```python
from build123d import *

# Parameters (mm, degrees)
F0_R     = 5
F0_R_2   = 4
F1_DEPTH = 2
F0_R_3   = 2.5
F2_DEPTH = 8.1
F0_R_4   = 1
F3_DEPTH = 12.5
F4_DEPTH = 12.5
F6_D     = 2
F6_DEPTH = 4
F6_TIP   = 0.600860619


with BuildPart() as f1:
    # F0 (on Front) → F1 (new body)
    with BuildSketch(Plane.XZ):
        Circle(F0_R)
        Circle(F0_R_2, mode=Mode.SUBTRACT)
    extrude(amount=F1_DEPTH)

    # F0 (on Front) → F2 (join)
    with BuildSketch(Plane.XZ):
        Circle(F0_R_2)
        Circle(F0_R_3, mode=Mode.SUBTRACT)
    extrude(amount=F2_DEPTH)

    # F0 (on Front) → F3 (join)
    with BuildSketch(Plane.XZ):
        Circle(F0_R_3)
        Circle(F0_R_4, mode=Mode.SUBTRACT)
    extrude(amount=F3_DEPTH)

    # F0 (on Front) → F4 (join)
    with BuildSketch(Plane.XZ):
        Circle(F0_R_4)
    extrude(amount=F4_DEPTH)

    # F6
    with Locations(Plane.XZ.offset(12.5)):
        with Locations((0, 0)):
            Hole(F6_D / 2, depth=F6_DEPTH)
            with Locations((0, 0, -(F6_DEPTH + F6_TIP / 2))):  # 118° drill point
                Cone(0, F6_D / 2, F6_TIP, mode=Mode.SUBTRACT)


solid = f1.part
```
CAD build for the part. Positions are in the model's coordinates, mm. A direction names the side the tool comes from. Round coordinates to 2 decimals unless told otherwise and drop trailing zeros. Order: outer loops, then holes, each group sorted by start corner. A loop starts at its lowest first (then second) coordinate and runs counter-clockwise, first axis right, second up. Notation, with made-up numbers: (73, 9.25) -> (86, 9.25) arc R20 ccw to (86, 27.25) -> close; hole circle Ø4 at (-26, -32). An arc over 180 degrees is marked (long way). One line per question, with ' | ' between items.
Q1. Slice it at A-A (x = 3.75). Write the cut outline in (y, z), then the cut area to 3 significant figures.
Completed:
outline: (-8.1, -1.39) -> (-2, -1.39) -> (-2, -3.31) -> (0, -3.31) -> (0, 3.31) -> (-2, 3.31) -> (-2, 1.39) -> (-8.1, 1.39) -> close | area: 30.2 mm^2
Q2. Slice it at C-C (z = -3.75). Write the cut outline in (x, y).
Completed:
outline: (-3.31, -2) -> (-1.39, -2) -> (-1.39, -8.1) -> (1.39, -8.1) -> (1.39, -2) -> (3.31, -2) -> (3.31, 0) -> (-3.31, 0) -> close
Q3. Which spindle directions (+Z, -Z, +X, -X, +Y, -Y) get a long thin tool onto all of the face, cutting with end or side? Do faces 5 (the cylindrical face through (-0.867, -5.007, -3.905)), 6 (the flat face through (0, 0, 0)). Say none if no direction does.
Completed:
face 5: -Y | face 6: +Z, -Z, +X, -X, +Y
Q4. Probe probe 1 along Z at (x, y) = (0, -10.3); probe 2 along Y at (x, z) = (-2, 3.5); probe 3 along Y at (x, z) = (3.25, 2). List the from-to ranges inside material, lowest first.
Completed:
probe 1: z = -2.5 to -1, 1 to 2.5 | probe 2: y = -2 to 0 | probe 3: y = -8.1 to 0
Q5. Two-plate mould, pull along X, no slides. Class faces 1 (the flat face through (2, -8.1, 2)), 2 (the cylindrical face through (-0.54, -10.27, -2.44)), 3 (the cylindrical face through (0, -10, -1)), 4 (the conical face through (-0.038, -8.003, -0.17)): released by +X, released by -X, zero draft, split by the parting line, or undercut.
Completed:
face 1: zero draft | face 2: split by the parting line | face 3: undercut | face 4: undercut
Q6. Drop flat-ended pins along their axis: pin 1 (2.5 mm diameter, centred on x = 0, z = 0, fed in from -Y); pin 2 (3 mm diameter, centred on y = -10.5, z = -3.5, fed in from -X); pin 3 (2 mm diameter, centred on x = 2, y = -4, fed in from -Z). Give the stop position or say it passes through.
Completed:
pin 1: stops at y = -12.5 | pin 2: stops at x = -1.5 | pin 3: stops at z = -3.87
Q7. Slice it at D-D (y = -10). Write the cut outline in (x, z).
Completed:
outline: circle Ø5 at (0, 0); hole circle Ø2 at (0, 0)
Q8. Slice it at B-B (y = -5). Write the cut outline in (x, z), then the cut area to 3 significant figures.
Completed:
outline: circle Ø8 at (0, 0) | area: 50.3 mm^2
